Verification items for this drawing (mm, ordinates from the low corner). A direction names the side the tool comes from. Give positions to 0.01 mm unless a question says otherwise; leave off trailing zeros. Loops run counter-clockwise (first coordinate to the right, second up) from the corner with the lowest first, then second, coordinate; pieces in that order, holes last. Notation, with made-up numbers: M 50.25,58 L 97.25,58 A11 cw 97.25,75 Z; hole C 1,0 d11. An arc over 180 degrees is marked long. Put each result on its own line as item: value. Start each with the question number.
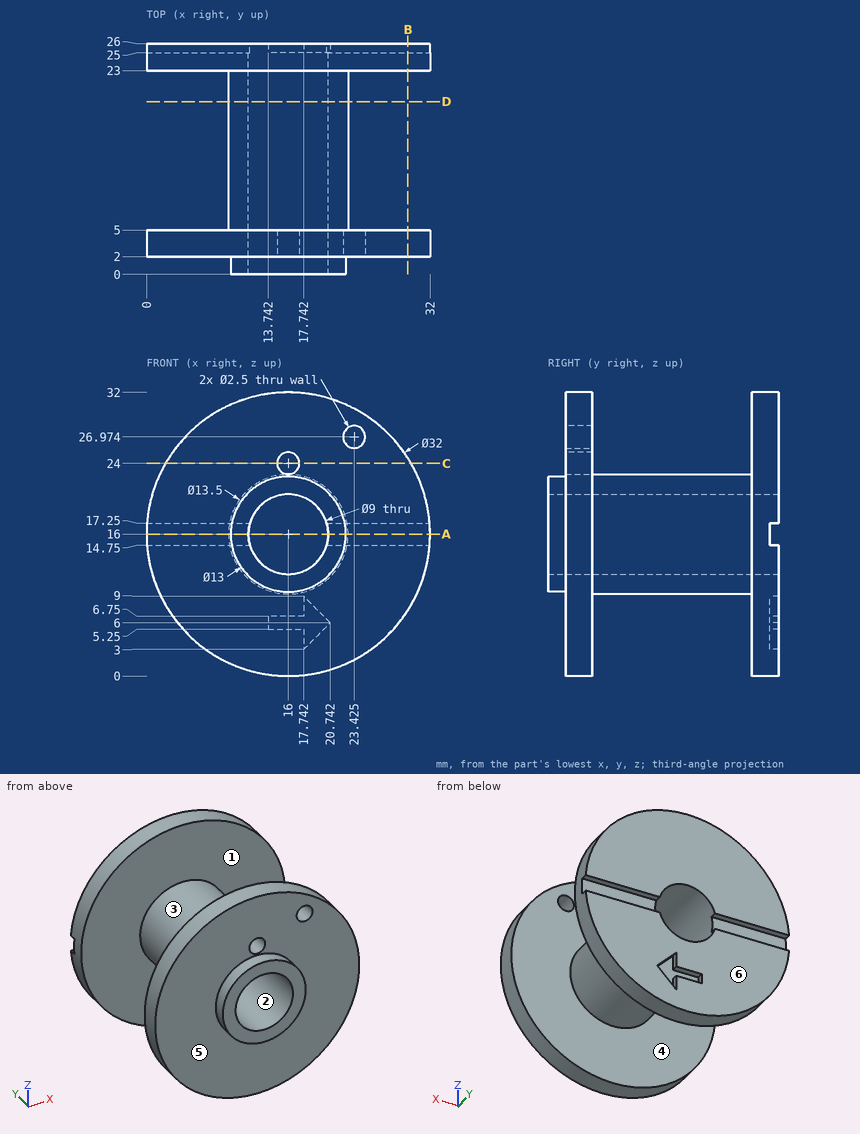
Q1. Scan lines: L1, parallel to Y at x = 21, z = 7.5; L2, parallel to Z at x = 16, y = 11.75; L3, parallel to Z at x = 12.5, y = 20. Record each from-to range of solid material in increasing order.
Q2. Set-up check for the marked faces 1 and 2: record each of +Z, -Z, +X, -X, +Y, -Y from which the full face is reachable in a straight line by a thin tool's end or side.
Q3. Release check for a two-part mould opening along Y. For the marked faces 3, 4, 5 and 6 record: pulls with the +Y half, pulls with the -Y half, needs draft (parallel to the pull), parting line crosses it, or undercut.
Q4. Cross-section at B-B, the plane x = 29.5. Record the boundary of the cut face in (y, z).
Q5. Cross-section at A-A, the plane z = 16. Record the boundary of the cut face in (x, y).
Q6. Cross-section at D-D, the plane y = 19.5. Record the boundary of the cut face in (x, z).
Q7. Cross-section at C-C, the plane z = 24. Record the boundary of the cut face in (x, y), then the cut area to 3 significant figures.
Q8. Go/stop test with flat-tipped pins: pin 1 (5 mm diameter, centred on x = 18.5, y = 6, fed in from -Z); pin 2 (6 mm diameter, centred on x = 17, z = 27.5, fed in from -Y); pin 3 (3 mm diameter, centred on y = 20, z = 23.5, fed in from +X) (1 decimal). Record where each tip stops, or that it passes through.
Ans:
1. L1: y = 2 to 5, 23 to 26
1. L2: z = 9.25 to 11.5, 20.5 to 22.75
1. L3: z = 10.23 to 13.17, 18.83 to 21.77
2. face 1: none
2. face 2: +Y, -Y
3. face 3: undercut
3. face 4: undercut
3. face 5: pulls with the -Y half
3. face 6: pulls with the +Y half
4. outline: M 2,7.41 L 5,7.41 L 5,24.59 L 2,24.59 Z; M 23,7.41 L 26,7.41 L 26,14.75 L 25,14.75 L 25,17.25 L 26,17.25 L 26,24.59 L 23,24.59 Z
5. outline: M 0,2 L 9.5,2 L 9.5,0 L 11.5,0 L 11.5,25 L 0,25 L 0,23 L 9.25,23 L 9.25,5 L 0,5 Z; M 20.5,0 L 22.5,0 L 22.5,2 L 32,2 L 32,5 L 22.75,5 L 22.75,23 L 32,23 L 32,25 L 20.5,25 Z
6. outline: C 16,16 d13.5; hole C 16,16 d9
7. outline: M 2.14,2 L 14.75,2 L 14.75,5 L 2.14,5 Z; M 2.14,23 L 29.86,23 L 29.86,26 L 2.14,26 Z; M 17.25,2 L 29.86,2 L 29.86,5 L 17.25,5 Z
7. area: 159 mm^2
8. pin 1: stops at z = 0
8. pin 2: stops at y = 2
8. pin 3: stops at x = 19.1
